Input: dimensioned drawing with shaded views. Units: mm. Origin: part minimum x, y, z. A direction names the side the tool comes from. Coordinates: 2 decimals unless noted, no trailing zeros. Loops run counter-clockwise (first coordinate to the right, second up) from the corner with the lowest first, then second, coordinate; pieces in that order, holes last.
Item 1: Pull-direction query (Z, two-part tool) for the marked faces 3, 4 and 5; classes: +Z half, -Z half, draft (parallel to the pull), parting line (faces both ways), or undercut.
Item 2: Section query A-A, the plane x = 18. Return the cut outline in (y, z) (1 decimal).
Item 3: Reachability of the marked faces 1 and 2 from +Z, -Z, +X, -X, +Y, -Y: full face, straight path, thin tool, end or side. Return the list, or none.
Item 4: Section query D-D, the plane z = 44. Return the cut outline in (x, y), then the cut area to 3 significant figures.
Item 5: Section query C-C, the plane z = 26. Return the cut outline in (x, y) (1 decimal), then the cut area to 3 significant figures.
Item 6: Pin query (flat end, axial travel): pin 1 Ø1 at (x, y) = (23, 4.5) entering from -Z; pin 2 Ø5 at (x, y) = (28.5, 2) entering from -Z; pin 3 Ø3 at (y, z) = (7, 40) entering from +X (1 decimal). Return the tip coordinate at first contact, or that it passes through.
Item 7: Line query: probe 1 along X at (y, z) = (6, 24) (1 decimal); probe 2 along Z at (x, y) = (17, 7.75) (1 decimal); probe 3 along Z at (x, y) = (26, 7) (1 decimal). Output: solid intervals per line, ascending.
Item 8: Section query B-B, the plane y = 2.25. Return the cut outline in (x, z) (1 decimal), then the cut area to 3 significant figures.
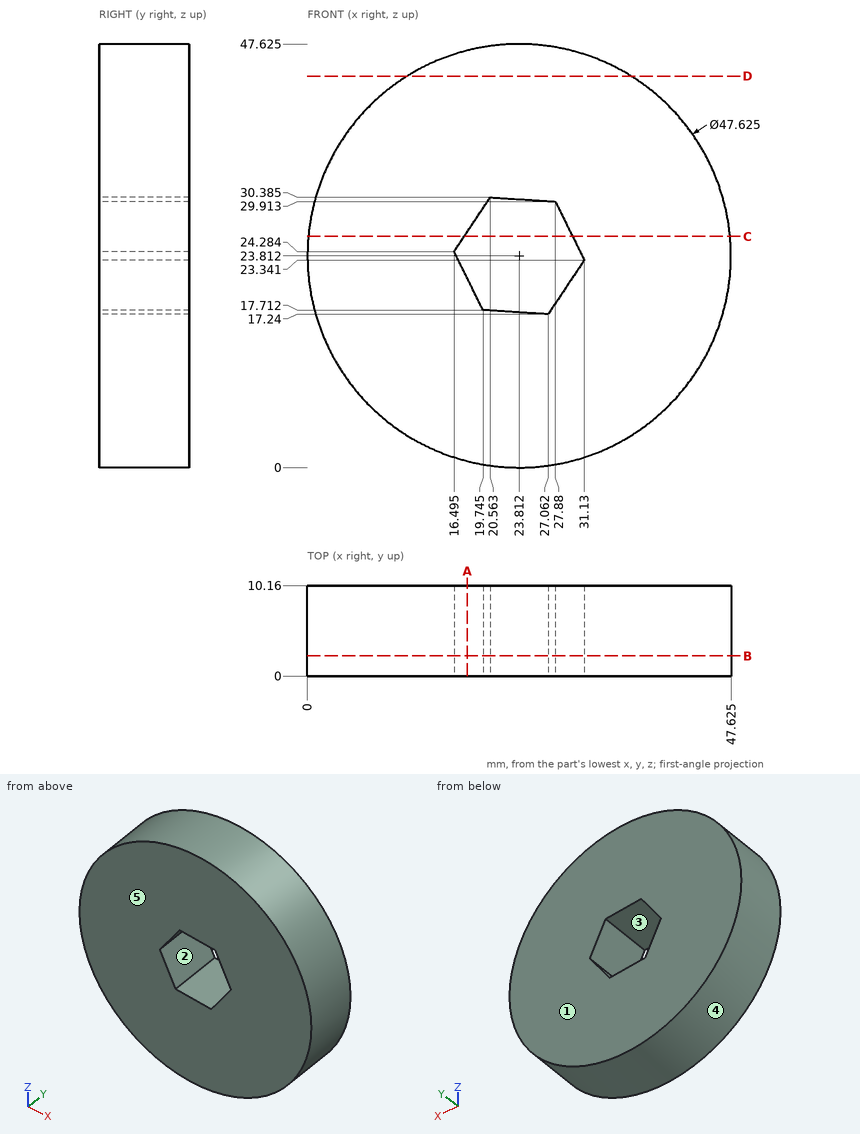
Verdict:
1. face 3: undercut
1. face 4: parting line
1. face 5: draft
2. outline: (0, 0.7) - (10.2, 0.7) - (10.2, 21.2) - (0, 21.2) - close; (0, 26.5) - (10.2, 26.5) - (10.2, 46.9) - (0, 46.9) - close
3. face 1: +Z, -Z, +X, -X, +Y
3. face 2: +Y, -Y
4. outline: (11.18, 0) - (36.44, 0) - (36.44, 10.16) - (11.18, 10.16) - close
4. area: 257 mm2
5. outline: (0.1, 0) - (17.6, 0) - (17.6, 10.2) - (0.1, 10.2) - close; (29.8, 0) - (47.5, 0) - (47.5, 10.2) - (29.8, 10.2) - close
5. area: 358 mm2
6. pin 1: stops at z = 0
6. pin 2: stops at z = 0.1
6. pin 3: stops at x = 42.6
7. probe 1: x = 0 to 16.6, 30.8 to 47.6
7. probe 2: z = 1 to 23.3, 25 to 46.6
7. probe 3: z = 0.1 to 17.3, 30 to 47.5
8. outline: circle Ø47.6 at (23.8, 23.8); hole (16.5, 24.3) - (19.7, 17.7) - (27.1, 17.2) - (31.1, 23.3) - (27.9, 29.9) - (20.6, 30.4) - close
8. area: 1,640 mm2
